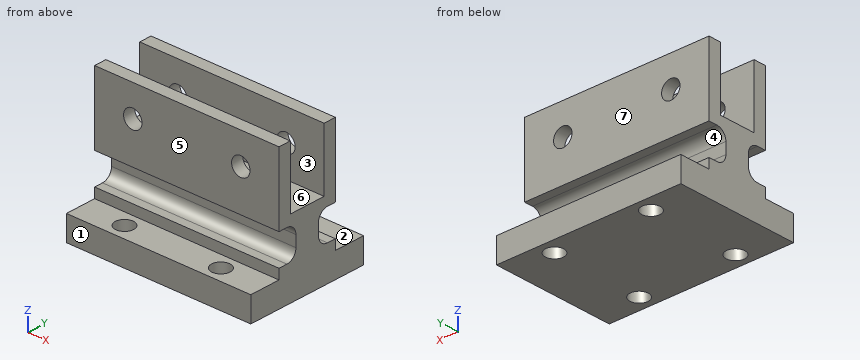
from build123d import *

# Parameters (mm, degrees)
F1_DEPTH = 7.5
F2_R     = 0.75
F3_DEPTH = 7.501
F4_R     = 0.75
F5_DEPTH = 2.001


with BuildPart() as f1:
    # F0 (on Right) → F1 (new body, symmetric)
    with BuildSketch(Plane.YZ):
        with BuildLine():
            Line((-1.5, -2.5), (-1.5, 2.5))
            Line((-1.5, 2.5), (-2.5, 2.5))
            Line((-2.5, 2.5), (-2.5, -3.3))
            Line((-2.5, -3.3), (-1.8, -3.3))
            ThreePointArc((-1.8, -3.3), (-1.234315, -3.534315), (-1, -4.1))
            Line((-1, -4.1), (-1, -5))
            ThreePointArc((-1, -5), (-1.234315, -5.565685), (-1.8, -5.8))
            Line((-1.8, -5.8), (-2.5, -5.8))
            Line((-2.5, -5.8), (-2.5, -6.6))
            Line((-2.5, -6.6), (2.5, -6.6))
            Line((2.5, -6.6), (2.5, -5.8))
            Line((2.5, -5.8), (1.8, -5.8))
            ThreePointArc((1.8, -5.8), (1.234315, -5.565685), (1, -5))
            Line((1, -5), (1, -4.1))
            ThreePointArc((1, -4.1), (1.234315, -3.534315), (1.8, -3.3))
            Line((1.8, -3.3), (2.5, -3.3))
            Line((2.5, -3.3), (2.5, 2.5))
            Line((2.5, 2.5), (1.5, 2.5))
            Line((1.5, 2.5), (1.5, -2.5))
            Line((1.5, -2.5), (-1.5, -2.5))
        make_face()
        Polygon((2.5, -6.6), (-2.5, -6.6), (-5, -6.6), (-5, -8.6), (5, -8.6), (5, -6.6), align=None)
    extrude(amount=F1_DEPTH, both=True)

    # F2 (on face) → F3 (cut, through all)
    with BuildSketch(Plane(origin=(0, 2.5, 0), x_dir=(-1, 0, 0), z_dir=(0, 1, 0))):
        with Locations((-4.395362, 0)):
            Circle(F2_R)
        with Locations((4.395362, 0)):
            Circle(F2_R)
    extrude(amount=-F3_DEPTH, mode=Mode.SUBTRACT)

    # F4 (on face) → F5 (cut, through all)
    with BuildSketch(Plane.XY.offset(-6.6)):
        with Locations((-3.921103, -3.75)):
            Circle(F4_R)
        with Locations((3.921103, -3.75)):
            Circle(F4_R)
        with Locations((3.921103, 3.75)):
            Circle(F4_R)
        with Locations((-3.921103, 3.75)):
            Circle(F4_R)
    extrude(amount=-F5_DEPTH, mode=Mode.SUBTRACT)


solid = f1.part
The model under review builds one solid part; all positions refer to its coordinate system, in mm. Face numbers are marked on the shaded views. A direction names the side the tool comes from. Give positions to 0.01 mm unless a question says otherwise; leave off trailing zeros. Order: outer loops, then holes, each group sorted by start corner. A loop starts at its lowest first (then second) coordinate and runs counter-clockwise, first axis right, second up. Notation, with made-up numbers: (88, 42) -> (112, 42) arc R26 ccw to (112, 69) -> close; hole circle Ø9 at (57.25, 3.25). An arc over 180 degrees is marked (long way). Write item = value, one per line. Start each with the question number.
(1) For pin 1 Ø0.6 at (x, z) = (-2, -6) entering from +Y; pin 2 Ø1 at (y, z) = (-1.5, -3.5) entering from +X; pin 3 Ø1.2 at (x, z) = (-4.4, 0) entering from -Y; pin 4 Ø0.7 at (x, z) = (3.5, -4.5) entering from +Y, all flat-tipped, find the tip position at first contact; note any pin that passes through.
(2) Tool access review of the marked faces 4, 5, 6 and 7: name each direction out of +Z, -Z, +X, -X, +Y, -Y from which nothing blocks a thin tool from reaching the whole face with its end or side.
(3) For L1, parallel to X at y = -4, z = -8; L2, parallel to Y at x = -3.5, z = 0; L3, parallel to Y at x = 4.5, z = -7.25, list the stretches that pass through material, from the lowest coordinate up. Write a range as from..to.
(4) Take a section at A-A (z = 1.5). Write out the cut boundary in (x, y), plus the area to 3 significant figures.
(5) Take a section at C-C (x = -2.5). Write out the cut boundary in (y, z).
(6) Draft analysis for pull direction Y (two halves, no side actions). For the marked faces 1, 2 and 3, state which applies: +Y half, -Y half, draft (parallel to the pull), parting line (faces both ways), or undercut.
(7) Take a section at D-D (y = -1.25). Write out the cut boundary in (x, z), plus the area to 3 significant figures.
(8) Take a section at B-B (y = 3.75). Write out the cut boundary in (x, z), plus the area to 3 significant figures.
Returned:
q1.pin_1 = 2.5
q1.pin_2 = 7.5
q1.pin_3 = through
q1.pin_4 = 1
q2.face_4 = +X, -X, +Y
q2.face_5 = +Z, +X, -X, -Y
q2.face_6 = +Z, +X, -X
q2.face_7 = +Z, +X, -X, +Y
q3.L1 = -7.5..-4.63, -3.21..3.21, 4.63..7.5
q3.L2 = -2.5..-1.5, 1.5..2.5
q3.L3 = -5..-4.23, -3.27..3.27, 4.23..5
q4.outline = (-7.5, -2.5) -> (7.5, -2.5) -> (7.5, -1.5) -> (-7.5, -1.5) -> close; (-7.5, 1.5) -> (7.5, 1.5) -> (7.5, 2.5) -> (-7.5, 2.5) -> close
q4.area = 30.0 mm²
q5.outline = (-5, -8.6) -> (5, -8.6) -> (5, -6.6) -> (2.5, -6.6) -> (2.5, -5.8) -> (1.8, -5.8) arc R0.8 cw to (1, -5) -> (1, -4.1) arc R0.8 cw to (1.8, -3.3) -> (2.5, -3.3) -> (2.5, 2.5) -> (1.5, 2.5) -> (1.5, -2.5) -> (-1.5, -2.5) -> (-1.5, 2.5) -> (-2.5, 2.5) -> (-2.5, -3.3) -> (-1.8, -3.3) arc R0.8 cw to (-1, -4.1) -> (-1, -5) arc R0.8 cw to (-1.8, -5.8) -> (-2.5, -5.8) -> (-2.5, -6.6) -> (-5, -6.6) -> close
q6.face_1 = -Y half
q6.face_2 = draft
q6.face_3 = undercut
q7.outline = (-7.5, -8.6) -> (7.5, -8.6) -> (7.5, -5.58) -> (-7.5, -5.58) -> close; (-7.5, -3.52) -> (7.5, -3.52) -> (7.5, -2.5) -> (-7.5, -2.5) -> close
q7.area = 60.6 mm²
q8.outline = (-7.5, -8.6) -> (-4.67, -8.6) -> (-4.67, -6.6) -> (-7.5, -6.6) -> close; (-3.17, -8.6) -> (3.17, -8.6) -> (3.17, -6.6) -> (-3.17, -6.6) -> close; (4.67, -8.6) -> (7.5, -8.6) -> (7.5, -6.6) -> (4.67, -6.6) -> close
q8.area = 24.0 mm²
